Check sheet for the modelled part. Datum: model origin and axes. Units: mm. A direction names the side the tool comes from. Round coordinates to 2 decimals unless told otherwise and drop trailing zeros. Write each loop counter-clockwise with the first axis right and the second up, starting at its lowest first coordinate (ties: lowest second). Pieces come first, ordered by that corner, then holes.
from build123d import *

# Parameters (mm, degrees)
BOSS_EXTRUDE1_DEPTH = 20
FILLET1_R           = 10


with BuildPart() as part:
    # Sketch1 → Boss-Extrude1 (new body)
    with BuildSketch(Plane.XY):
        Polygon((0, 0), (0, 20), (3, 20), (3, 0), (7, 0), (7, 20), (11.5, 20), (11.5, 24), (-8.5, 24), (-8.5, 20), (-4, 20), (-4, 0), align=None)
    extrude(amount=BOSS_EXTRUDE1_DEPTH)

    # Fillet1
    # the kernel refuses this fillet: 10 mm, written as the material it adds along each edge
    with BuildSketch(Plane(origin=(-4, 20, 0), x_dir=(-1.0, -1.533193325383024e-12, 0), z_dir=(0, 0, 1))) as fillet1_piece_1:
        with BuildLine():
            CenterArc((10, 8.351646544), FILLET1_R, 180, 56.632987031)
            Line((0, 8.351646544), (-0.2, 8.351646544))
            Line((-0.2, 8.351646544), (-0.2, 0))
            Line((-0.2, 0), (0, -0.2))
            ThreePointArc((0, -0.2), (2.25, -0.2), (4.39, -0.167032931))
            Line((4.39, -0.167032931), (4.5, 0))
        make_face()
    extrude(amount=20)
    with BuildSketch(Plane(origin=(7, 20, 0), x_dir=(0, -1, 0), z_dir=(0, 0, 1))) as fillet1_piece_2:
        with BuildLine():
            CenterArc((8.351646544, 10), FILLET1_R, 213.367012969, 56.632987031)
            Line((0, 4.5), (-0.167032931, 4.39))
            ThreePointArc((-0.167032931, 4.39), (-0.2, 2.25), (-0.2, 0))
            Line((-0.2, 0), (0, -0.2))
            Line((0, -0.2), (8.351646544, -0.2))
            Line((8.351646544, -0.2), (8.351646544, 0))
        make_face()
    extrude(amount=20)


solid = part.part
1. Sectioned sample at C-C, the plane y = 19.5. Enter the section's corners in (x, z).
2. Sectioned sample at A-A, the plane y = 3. Enter the section's corners in (x, z).
3. Release check for a two-part mould opening along X. For faces 1 (the flat face through (-8.5, 22, 10)), 2 (the flat face through (0, 10, 10)), 3 (the flat face through (4, 14, 0)) record: released by +X, released by -X, zero draft, split by the parting line, or undercut.
4. Sectioned sample at D-D, the plane x = 1.75. Enter the section's corners in (y, z), plus the area to 3 significant figures.
5. Go/stop test with flat-tipped pins: pin 1 (2 mm diameter, centred on y = 9.5, z = 6, fed in from +X); pin 2 (3.5 mm diameter, centred on y = 4.5, z = 12.5, fed in from -X); pin 3 (0.9 mm diameter, centred on x = 1.5, z = 7, fed in from -Y). Record where each tip stops, or that it passes through.
6. Scan lines: line 1 along X through (y, z) = (7.5, 16.25); line 2 along X through (y, z) = (17, 12); line 3 along Y through (x, z) = (2.5, 2.5). Record each from-to range of solid material in increasing order.
7. Sectioned sample at B-B, the plane z = 18.25. Enter the section's corners in (x, y).
8. Set-up check for faces 4 (the flat face through (11.5, 22, 10)), 5 (the flat face through (3, 10, 10)), 6 (the flat face through (7, 6, 10)), 7 (the flat face through (-4, 6, 10)): record each of +Z, -Z, +X, -X, +Y, -Y from which the full face is reachable in a straight line by a thin tool's end or side.
Computed values:
1. outline: (-7.81, 0) - (0, 0) - (0, 20) - (-7.81, 20) - close; (3, 0) - (10.81, 0) - (10.81, 20) - (3, 20) - close
2. outline: (-4, 0) - (0, 0) - (0, 20) - (-4, 20) - close; (3, 0) - (7, 0) - (7, 20) - (3, 20) - close
3. face 1: released by -X
3. face 2: undercut
3. face 3: zero draft
4. outline: (20, 0) - (24, 0) - (24, 20) - (20, 20) - close
4. area: 80.0 mm2
5. pin 1: stops at x = 7
5. pin 2: stops at x = -4
5. pin 3: stops at y = 20
6. line 1: x = -4 to 0, 3 to 7
6. line 2: x = -5.55 to 0, 3 to 8.55
6. line 3: y = 20 to 24
7. outline: (-8.5, 20) arc R10 cw to (-4, 11.65) - (-4, 0) - (0, 0) - (0, 20) - (3, 20) - (3, 0) - (7, 0) - (7, 11.65) arc R10 cw to (11.5, 20) - (11.5, 24) - (-8.5, 24) - close
8. face 4: +Z, -Z, +X, +Y, -Y
8. face 5: +Z, -Z, -Y
8. face 6: +Z, -Z, +X, -Y
8. face 7: +Z, -Z, -X, -Y
